Part model, mm, in its own coordinate system. Give positions to 0.01 mm unless a question says otherwise; leave off trailing zeros. Order: outer loops, then holes, each group sorted by start corner. A loop starts at its lowest first (then second) coordinate and runs counter-clockwise, first axis right, second up. Notation, with made-up numbers: (-31, 14) -> (10, 14) arc R8 ccw to (10, 25) -> close; hole circle Ø5 at (73, 37). An arc over 180 degrees is marked (long way). Write item = value, one per line. Start each with the question number.
(1) Saw through at B-B, the plane z = -1.5. List the corners of the cut face in (x, y), then the cut area to 3 significant figures.
(2) Flat gauge pins, fed straight in: pin 1 (4 mm diameter, centred on y = -34, z = 9.5, fed in from -X); pin 2 (19 mm diameter, centred on x = -78.5, y = -51, fed in from -Z); pin 3 (5 mm diameter, centred on x = -115.5, y = -69, fed in from +Z); pin 4 (2.5 mm diameter, centred on x = -114.9, y = -69, fed in from +Z). Where does each tip first touch, or does it go through?
(3) Saw through at A-A, the plane y = -69. List the corners of the cut face in (x, z).
(4) Saw through at C-C, the plane y = 0. State how many separate pieces and enclosed holes the cut face has, then the cut area to 3 significant figures.
(5) Probe line 1 along X through (y, z) = (0, 12.2); line 2 along Z through (x, y) = (-38, -25); line 3 along Y through (x, z) = (-18.5, 3). List the from-to ranges inside material, lowest first. Write a range as from..to.
(6) Saw through at D-D, the plane x = -35. List the corners of the cut face in (y, z), then the cut area to 3 significant figures.
from build123d import *

# Parameters (mm, degrees)
CROQUIS1_R              = 1.5
SALIENTE_EXTRUIR1_DEPTH = 10
CROQUIS2_W              = 45
CROQUIS2_H              = 10.081197804
CORTAR_EXTRUIR1_DEPTH   = 50
CROQUIS3_R              = 1.5
SALIENTE_EXTRUIR2_DEPTH = 10
CROQUIS4_W              = 25
CROQUIS4_H              = 10
CORTAR_EXTRUIR2_DEPTH   = 50
SALIENTE_EXTRUIR3_DEPTH = 10
CROQUIS7_W              = 22
CROQUIS7_H              = 10
CORTAR_EXTRUIR4_DEPTH   = 20
REDONDEO1_R             = 10


with BuildPart() as part:
    # Croquis1 → Saliente-Extruir1 (new body)
    with BuildSketch(Plane.XY):
        with BuildLine():
            Line((0, -5), (-10, -5))
            Line((-10, -5), (-90, -74))
            Line((-90, -74), (-114.8954508, -74))
            ThreePointArc((-114.8954508, -74), (-119.8954508, -69), (-114.8954508, -64))
            Line((-114.8954508, -64), (-94.556304917, -64))
            Line((-94.556304917, -64), (-10, 5))
            Line((-10, 5), (0, 5))
            ThreePointArc((0, 5), (5, 0), (0, -5))
        make_face()
        Circle(CROQUIS1_R, mode=Mode.SUBTRACT)
        with Locations((-114.8954508, -69)):
            Circle(CROQUIS1_R, mode=Mode.SUBTRACT)
    extrude(amount=SALIENTE_EXTRUIR1_DEPTH)

    # Croquis2 → Cortar-Extruir1 (cut)
    with BuildSketch(Plane(origin=(0, -64, 0), x_dir=(1, 0, 0), z_dir=(0, 1, 0))):
        with Locations((-119.8954508, 2.540598902)):
            Rectangle(CROQUIS2_W, CROQUIS2_H)
        with Locations((-119.8954508, -12.540598902)):
            Rectangle(CROQUIS2_W, CROQUIS2_H)
    extrude(amount=-CORTAR_EXTRUIR1_DEPTH, mode=Mode.SUBTRACT)

    # Croquis3 → Saliente-Extruir2 (add, symmetric)
    with BuildSketch(Plane.XY.offset(5)):
        with BuildLine():
            Line((0, 5), (-10, 5))
            Line((-10, 5), (-10, -5))
            Line((-10, -5), (0, -5))
            ThreePointArc((0, -5), (5, 0), (0, 5))
        make_face()
        Circle(CROQUIS3_R, mode=Mode.SUBTRACT)
    extrude(amount=SALIENTE_EXTRUIR2_DEPTH, both=True)

    # Croquis4 → Cortar-Extruir2 (cut)
    with BuildSketch(Plane(origin=(0, 5, 0), x_dir=(1, 0, 0), z_dir=(0, 1, 0))):
        with Locations((5, -5)):
            Rectangle(CROQUIS4_W, CROQUIS4_H)
    extrude(amount=-CORTAR_EXTRUIR2_DEPTH, mode=Mode.SUBTRACT)

    # Croquis5 → Saliente-Extruir3 (add, symmetric)
    with BuildSketch(Plane.XY.offset(5)):
        Polygon((-22.5, -5.200303819), (-17.266882634, -11.267686272), (-10, -5), (-10, 5), align=None)
    extrude(amount=SALIENTE_EXTRUIR3_DEPTH, both=True)

    # Croquis7 → Cortar-Extruir4 (cut)
    with BuildSketch(Plane(origin=(-6.446429036, 7.899800278, 0), x_dir=(0.7747758954984266, 0.6322359620858428, 0), z_dir=(-0.6322359620858428, 0.7747758954984267, 0))):
        with Locations((-6, -5)):
            Rectangle(CROQUIS7_W, CROQUIS7_H)
    extrude(amount=-CORTAR_EXTRUIR4_DEPTH, mode=Mode.SUBTRACT)

    # Redondeo1
    # the kernel refuses this fillet: 10 mm, written as the material it adds along each edge
    with BuildSketch(Plane(origin=(-17.266882634, -11.267686272, 0), x_dir=(0, 0, -1), z_dir=(-0.6531268480840459, 0.757248519517734, 0))) as redondeo1_piece_1_section:
        with BuildLine():
            CenterArc((10, 8.660254038), REDONDEO1_R, 180, 60)
            Line((0, 8.660254038), (-0.2, 8.660254038))
            Line((-0.2, 8.660254038), (-0.2, 0))
            Line((-0.2, 0), (0, -0.2))
            ThreePointArc((0, -0.2), (2.5, -0.2), (4.9, -0.173205081))
            Line((4.9, -0.173205081), (5, 0))
        make_face()
    redondeo1_piece_1 = extrude(amount=29.663040925, mode=Mode.PRIVATE)
    redondeo1_piece_1 = split(redondeo1_piece_1, bisect_by=Plane(origin=(-24.101226761, -6.506943775, -1.290515282), z_dir=(0.6322359620858427, -0.7747758954984267, 0)), keep=Keep.TOP, mode=Mode.PRIVATE)
    add(redondeo1_piece_1)
    with BuildSketch(Plane(origin=(-97.3954508, -64, 2.5), x_dir=(-1, 0, 0), z_dir=(0, -1, 0))) as redondeo1_piece_2:
        with BuildLine():
            CenterArc((6.614378278, 10), REDONDEO1_R, 228.590377891, 41.409622109)
            Line((0, 2.5), (-0.132287566, 2.35))
            ThreePointArc((-0.132287566, 2.35), (-0.2, 1.25), (-0.2, 0))
            Line((-0.2, 0), (0, -0.2))
            Line((0, -0.2), (6.614378278, -0.2))
            Line((6.614378278, -0.2), (6.614378278, 0))
        make_face()
    extrude(amount=10)
    with BuildSketch(Plane(origin=(-97.3954508, -64, 7.5), x_dir=(0, 0, 1), z_dir=(0, -1, 0))) as redondeo1_piece_3:
        with BuildLine():
            CenterArc((10, 6.614378278), REDONDEO1_R, 180, 41.409622109)
            Line((0, 6.614378278), (-0.2, 6.614378278))
            Line((-0.2, 6.614378278), (-0.2, 0))
            Line((-0.2, 0), (0, -0.2))
            ThreePointArc((0, -0.2), (1.25, -0.2), (2.35, -0.132287566))
            Line((2.35, -0.132287566), (2.5, 0))
        make_face()
    extrude(amount=10)
    with BuildSketch(Plane(origin=(-17.266882634, -11.267686272, 10), x_dir=(-0.757248519517734, -0.6531268480840459, 0), z_dir=(-0.6531268480840459, 0.757248519517734, 0))) as redondeo1_piece_4_section:
        with BuildLine():
            CenterArc((8.660254038, 10), REDONDEO1_R, 210, 60)
            Line((0, 5), (-0.173205081, 4.9))
            ThreePointArc((-0.173205081, 4.9), (-0.2, 2.5), (-0.2, 0))
            Line((-0.2, 0), (0, -0.2))
            Line((0, -0.2), (8.660254038, -0.2))
            Line((8.660254038, -0.2), (8.660254038, 0))
        make_face()
    redondeo1_piece_4 = extrude(amount=29.663040925, mode=Mode.PRIVATE)
    redondeo1_piece_4 = split(redondeo1_piece_4, bisect_by=Plane(origin=(-24.101226761, -6.506943775, 11.290515282), z_dir=(0.6322359620858427, -0.7747758954984267, 0)), keep=Keep.TOP, mode=Mode.PRIVATE)
    add(redondeo1_piece_4)
    with BuildSketch(Plane(origin=(-19.617619259, -2.848211077, 0), x_dir=(0, 0, 1), z_dir=(0.6322359620858428, -0.7747758954984266, 0))) as redondeo1_piece_5_section:
        with BuildLine():
            CenterArc((REDONDEO1_R, -REDONDEO1_R), REDONDEO1_R, 90, 90)
            Line((0, -REDONDEO1_R), (-REDONDEO1_R * 0.02, -REDONDEO1_R))
            Line((-REDONDEO1_R * 0.02, -REDONDEO1_R), (-REDONDEO1_R * 0.02, REDONDEO1_R * 0.02))
            Line((-REDONDEO1_R * 0.02, REDONDEO1_R * 0.02), (REDONDEO1_R, REDONDEO1_R * 0.02))
            Line((REDONDEO1_R, REDONDEO1_R * 0.02), (REDONDEO1_R, 0))
        make_face()
    redondeo1_piece_5 = extrude(amount=32.91390687, mode=Mode.PRIVATE)
    redondeo1_piece_5 = split(redondeo1_piece_5, bisect_by=Plane(origin=(-15.697629804, -5, 1.81207327), z_dir=(0, 1, 0)), keep=Keep.TOP, mode=Mode.PRIVATE)
    redondeo1_piece_5 = split(redondeo1_piece_5, bisect_by=Plane(origin=(-12.240787311, -6.932679056, 1.81207327), z_dir=(-0.6531268480840465, 0.7572485195177333, 0)), keep=Keep.TOP, mode=Mode.PRIVATE)
    add(redondeo1_piece_5)
    with BuildSketch(Plane(origin=(-19.617619259, -2.848211077, 0), x_dir=(0, 0, 1), z_dir=(0.6322359620858428, -0.7747758954984266, 0))) as redondeo1_piece_6_section:
        with BuildLine():
            CenterArc((REDONDEO1_R, -REDONDEO1_R), REDONDEO1_R, 90, 90)
            Line((0, -REDONDEO1_R), (-REDONDEO1_R * 0.02, -REDONDEO1_R))
            Line((-REDONDEO1_R * 0.02, -REDONDEO1_R), (-REDONDEO1_R * 0.02, REDONDEO1_R * 0.02))
            Line((-REDONDEO1_R * 0.02, REDONDEO1_R * 0.02), (REDONDEO1_R, REDONDEO1_R * 0.02))
            Line((REDONDEO1_R, REDONDEO1_R * 0.02), (REDONDEO1_R, 0))
        make_face()
    redondeo1_piece_6 = extrude(amount=32.91390687, mode=Mode.PRIVATE)
    redondeo1_piece_6 = split(redondeo1_piece_6, bisect_by=Plane(origin=(-7.753376127, -5, 0.000921207), z_dir=(0, 1, 0)), keep=Keep.TOP, mode=Mode.PRIVATE)
    redondeo1_piece_6 = split(redondeo1_piece_6, bisect_by=Plane(origin=(-8.357285081, -3.583158383, 0.000921207), z_dir=(0.6531268480840465, -0.7572485195177333, 0)), keep=Keep.TOP, mode=Mode.PRIVATE)
    add(redondeo1_piece_6)
    with BuildSketch(Plane(origin=(-19.617619259, -2.848211077, 0), x_dir=(0, 0, 1), z_dir=(0.6322359620858428, -0.7747758954984266, 0))) as redondeo1_piece_7_section:
        with BuildLine():
            CenterArc((REDONDEO1_R, -REDONDEO1_R), REDONDEO1_R, 90, 90)
            Line((0, -REDONDEO1_R), (-REDONDEO1_R * 0.02, -REDONDEO1_R))
            Line((-REDONDEO1_R * 0.02, -REDONDEO1_R), (-REDONDEO1_R * 0.02, REDONDEO1_R * 0.02))
            Line((-REDONDEO1_R * 0.02, REDONDEO1_R * 0.02), (REDONDEO1_R, REDONDEO1_R * 0.02))
            Line((REDONDEO1_R, REDONDEO1_R * 0.02), (REDONDEO1_R, 0))
        make_face()
    redondeo1_piece_7 = extrude(amount=32.91390687, mode=Mode.PRIVATE)
    redondeo1_piece_7 = split(redondeo1_piece_7, bisect_by=Plane(origin=(-14.976833445, -5, 2.906461965), z_dir=(0, -1, 0)), keep=Keep.TOP, mode=Mode.PRIVATE)
    redondeo1_piece_7 = split(redondeo1_piece_7, bisect_by=Plane(origin=(-13.639024157, -8.138658336, 2.906461965), z_dir=(-0.6531268480840465, 0.7572485195177333, 0)), keep=Keep.TOP, mode=Mode.PRIVATE)
    add(redondeo1_piece_7)
    with BuildSketch(Plane(origin=(-19.617619259, -2.848211077, 10), x_dir=(0, 0, -1), z_dir=(0.6322359620858428, -0.7747758954984266, 0))) as redondeo1_piece_8_section:
        with BuildLine():
            CenterArc((REDONDEO1_R, REDONDEO1_R), REDONDEO1_R, 180, 90)
            Line((0, REDONDEO1_R), (-REDONDEO1_R * 0.02, REDONDEO1_R))
            Line((-REDONDEO1_R * 0.02, REDONDEO1_R), (-REDONDEO1_R * 0.02, -REDONDEO1_R * 0.02))
            Line((-REDONDEO1_R * 0.02, -REDONDEO1_R * 0.02), (REDONDEO1_R, -REDONDEO1_R * 0.02))
            Line((REDONDEO1_R, -REDONDEO1_R * 0.02), (REDONDEO1_R, 0))
        make_face()
    redondeo1_piece_8 = extrude(amount=32.91390687, mode=Mode.PRIVATE)
    redondeo1_piece_8 = split(redondeo1_piece_8, bisect_by=Plane(origin=(-15.697629804, -5, 8.18792673), z_dir=(0, 1, 0)), keep=Keep.TOP, mode=Mode.PRIVATE)
    redondeo1_piece_8 = split(redondeo1_piece_8, bisect_by=Plane(origin=(-12.240787311, -6.932679056, 8.18792673), z_dir=(-0.6531268480840465, 0.7572485195177333, 0)), keep=Keep.TOP, mode=Mode.PRIVATE)
    add(redondeo1_piece_8)
    with BuildSketch(Plane(origin=(-19.617619259, -2.848211077, 10), x_dir=(0, 0, -1), z_dir=(0.6322359620858428, -0.7747758954984266, 0))) as redondeo1_piece_9_section:
        with BuildLine():
            CenterArc((REDONDEO1_R, REDONDEO1_R), REDONDEO1_R, 180, 90)
            Line((0, REDONDEO1_R), (-REDONDEO1_R * 0.02, REDONDEO1_R))
            Line((-REDONDEO1_R * 0.02, REDONDEO1_R), (-REDONDEO1_R * 0.02, -REDONDEO1_R * 0.02))
            Line((-REDONDEO1_R * 0.02, -REDONDEO1_R * 0.02), (REDONDEO1_R, -REDONDEO1_R * 0.02))
            Line((REDONDEO1_R, -REDONDEO1_R * 0.02), (REDONDEO1_R, 0))
        make_face()
    redondeo1_piece_9 = extrude(amount=32.91390687, mode=Mode.PRIVATE)
    redondeo1_piece_9 = split(redondeo1_piece_9, bisect_by=Plane(origin=(-7.753376127, -5, 9.999078793), z_dir=(0, 1, 0)), keep=Keep.TOP, mode=Mode.PRIVATE)
    redondeo1_piece_9 = split(redondeo1_piece_9, bisect_by=Plane(origin=(-8.357285081, -3.583158383, 9.999078793), z_dir=(0.6531268480840465, -0.7572485195177333, 0)), keep=Keep.TOP, mode=Mode.PRIVATE)
    add(redondeo1_piece_9)
    with BuildSketch(Plane(origin=(-19.617619259, -2.848211077, 10), x_dir=(0, 0, -1), z_dir=(0.6322359620858428, -0.7747758954984266, 0))) as redondeo1_piece_10_section:
        with BuildLine():
            CenterArc((REDONDEO1_R, REDONDEO1_R), REDONDEO1_R, 180, 90)
            Line((0, REDONDEO1_R), (-REDONDEO1_R * 0.02, REDONDEO1_R))
            Line((-REDONDEO1_R * 0.02, REDONDEO1_R), (-REDONDEO1_R * 0.02, -REDONDEO1_R * 0.02))
            Line((-REDONDEO1_R * 0.02, -REDONDEO1_R * 0.02), (REDONDEO1_R, -REDONDEO1_R * 0.02))
            Line((REDONDEO1_R, -REDONDEO1_R * 0.02), (REDONDEO1_R, 0))
        make_face()
    redondeo1_piece_10 = extrude(amount=32.91390687, mode=Mode.PRIVATE)
    redondeo1_piece_10 = split(redondeo1_piece_10, bisect_by=Plane(origin=(-14.976833445, -5, 7.093538035), z_dir=(0, -1, 0)), keep=Keep.TOP, mode=Mode.PRIVATE)
    redondeo1_piece_10 = split(redondeo1_piece_10, bisect_by=Plane(origin=(-13.639024157, -8.138658336, 7.093538035), z_dir=(-0.6531268480840465, 0.7572485195177333, 0)), keep=Keep.TOP, mode=Mode.PRIVATE)
    add(redondeo1_piece_10)


solid = part.part
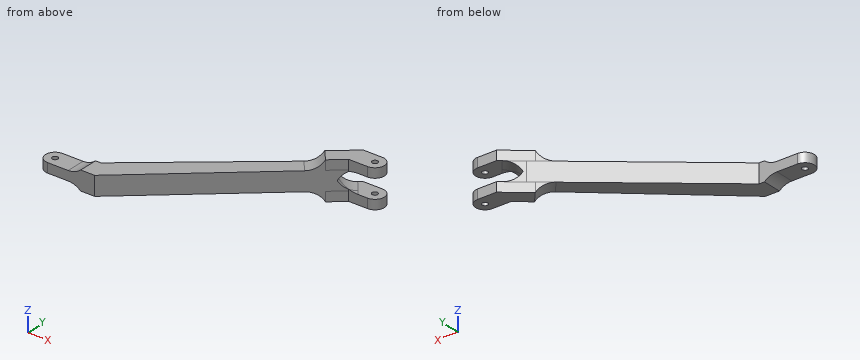
Results list:
q1.outline = (-25.13, -7.35) -> (-19.84, -13.48) -> (-10, -5) -> (0, -5) arc R5 ccw to (0, 5) -> (-10, 5) -> close; hole circle Ø3 at (0, 0)
q1.area = 260 mm^2
q2.pin_1 = -60.24
q2.pin_2 = 0
q2.pin_3 = 7.5
q2.pin_4 = through
q3.outline = (-119.9, 2.5) -> (-116.4, 2.5) -> (-116.4, 7.5) -> (-119.9, 7.5) -> close; (-113.4, 2.5) -> (-104.01, 2.5) arc R10 cw to (-97.4, 0) -> (-84.2, 0) -> (-84.2, 10) -> (-97.4, 10) arc R10 cw to (-104.01, 7.5) -> (-113.4, 7.5) -> close
q4.separate_pieces = 4
q4.enclosed_holes = 0
q4.area = 189 mm^2
q5.line_1 = -16.13..-1.5, 1.5..5
q5.line_2 = 0..10
q5.line_3 = -12.33..-1.94
q6.outline = (-26.56, 0) -> (-15.4, 0) -> (-15.4, 10) -> (-26.56, 10) -> close
q6.area = 112 mm^2
